Build history of the part. All positions in model axes, mm. Face numbers are marked on the shaded views. A direction names the side the tool comes from. Give positions to 0.01 mm unless a question says otherwise; leave off trailing zeros. Order: outer loops, then holes, each group sorted by start corner. A loop starts at its lowest first (then second) coordinate and runs counter-clockwise, first axis right, second up. Notation, with made-up numbers: M -14.5,54 L -8.5,54 A20 cw -8.5,61 Z; hole C -14,-40 d5. An arc over 180 degrees is marked long. Answer as CSV lines item,"result".
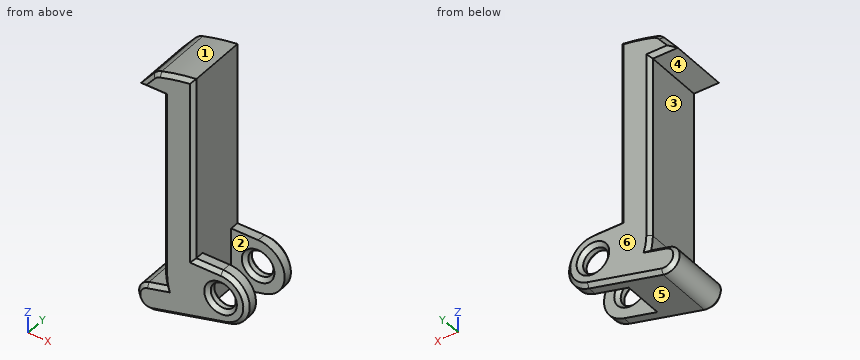
from build123d import *

# Parameters (mm, degrees)
SKETCH1_R           = 1.65
BOSS_EXTRUDE1_DEPTH = 8.6
SKETCH2_W           = 7.05
SKETCH2_H           = 5.3
CUT_EXTRUDE1_DEPTH  = 28.041671481
CHAMFER1_SIZE       = 0.5
CUT_EXTRUDE2_DEPTH  = 36.823034653
FILLET1_R           = 2
CHAMFER2_SIZE       = 0.5


with BuildPart() as part:
    # Sketch1 → Boss-Extrude1 (new body)
    with BuildSketch(Plane(origin=(0, 0, 0), x_dir=(1, 0, 0), z_dir=(0, 1, 0))):
        with BuildLine():
            Line((4.41627224, 31.391101946), (-5.369479089, 33.890916124))
            ThreePointArc((-5.369479089, 33.890916124), (-7.498166182, 32.628501271), (-6.235751329, 30.499814178))
            Line((-6.235751329, 30.499814178), (-3.76509134, 29.868672975))
            ThreePointArc((-3.76509134, 29.868672975), (-3.941042638, 28.941690072), (-4, 28))
            Line((-4, 28), (-4, 4))
            Line((-4, 4), (-7.3, 4))
            Line((-7.3, 4), (-4, 0))
            Line((-4, 0), (0, 0))
            Line((0, 0), (0, 24.5))
            Line((0, 24.5), (3.55, 24.5))
            ThreePointArc((3.55, 24.5), (7.022668773, 27.563454934), (4.41627224, 31.391101946))
        make_face()
        with Locations(Location((3.55, 28, 0), (0, 0, 90))):
            Circle(SKETCH1_R, mode=Mode.SUBTRACT)
    extrude(amount=BOSS_EXTRUDE1_DEPTH)

    # Sketch2 → Cut-Extrude1 (cut, through all)
    with BuildSketch(Plane.XY.offset(-24.5)):
        with Locations((3.525, 4.3)):
            Rectangle(SKETCH2_W, SKETCH2_H)
    extrude(amount=-CUT_EXTRUDE1_DEPTH, mode=Mode.SUBTRACT)

    # Chamfer1
    chamfer1_edges = [part.edges().sort_by_distance(p)[0] for p in [
        (3.55, 0, -26.35),
        (3.55, 8.6, -26.35),
        (3.55, 6.95, -26.35),
        (3.55, 1.65, -26.35),
    ]]
    chamfer(chamfer1_edges, length=CHAMFER1_SIZE)

    # Sketch3 → Cut-Extrude2 (cut, through all)
    with BuildSketch(Plane(origin=(0, 0, 0), x_dir=(1, 0, 0), z_dir=(0, 1, 0))):
        with BuildLine():
            Line((0, 0.225956362), (0, 0))
            Line((0, 0), (-4, 0))
            Line((-4, 0), (-5.140926966, 1.382941776))
            ThreePointArc((-5.140926966, 1.382941776), (-2.597741622, 0.683241903), (0, 0.225956362))
        make_face()
    extrude(amount=CUT_EXTRUDE2_DEPTH, mode=Mode.SUBTRACT)

    # Fillet1
    fillet1_edges = [part.edges().sort_by_distance(p)[0] for p in [
        (-5.140926966, 4.3, -1.382941776),
    ]]
    fillet(fillet1_edges, radius=FILLET1_R)

    # Chamfer2
    chamfer2_edges = [part.edges().sort_by_distance(p)[0] for p in [
        (-5.083597869, 8.6, -1.448008405),
        (-6.409042622, 0, -2.920051663),
        (-5.65, 0, -4),
        (-4, 0, -16),
        (-3.941042638, 0, -28.941690072),
        (7.022668773, 8.6, -27.563454934),
        (-5.000421335, 0, -30.184243577),
        (-7.498166182, 0, -32.628501271),
        (-0.476603424, 0, -32.641009035),
        (7.022668773, 0, -27.563454934),
        (1.775, 0, -24.5),
        (-0.476603424, 8.6, -32.641009035),
        (-7.498166182, 8.6, -32.628501271),
        (-5.000421335, 8.6, -30.184243577),
        (-3.941042638, 8.6, -28.941690072),
        (-4, 8.6, -16),
        (-5.65, 8.6, -4),
        (-6.409042622, 8.6, -2.920051663),
        (0, 0, -12.362978181),
        (0, 8.6, -12.362978181),
        (-2.297358874, 0, -0.617370576),
        (-2.297358874, 8.6, -0.617370576),
        (1.775, 8.6, -24.5),
        (-5.083597869, 0, -1.448008405),
    ]]
    chamfer(chamfer2_edges, length=CHAMFER2_SIZE)


solid = part.part
Item 1: Pull direction Z, two halves, no side cores. Call the marked faces 3, 4, 5 and 6: released by +Z, released by -Z, zero draft, split by the parting line, or undercut.
Geometry says:
face 3,"undercut"
face 4,"undercut"
face 5,"released by -Z"
face 6,"zero draft"
Item 2: Drop flat-ended pins along their axis: pin 1 (1 mm diameter, centred on x = 1.5, y = 1, fed in from +Z); pin 2 (3 mm diameter, centred on x = 3.55, z = -28, fed in from -Y); pin 3 (5 mm diameter, centred on x = -5, y = 3.5, fed in from +Z); pin 4 (4 mm diameter, centred on y = 5, z = -17, fed in from -X). Give the stop position or say it passes through.
Geometry says:
pin 1,"stops at z = -24.5"
pin 2,"passes through"
pin 3,"stops at z = -0.66"
pin 4,"stops at x = -4"
Item 3: Band-saw the part on A-A (z = -4.5). Give the cut face in (x, y).
Geometry says:
outline,"M -4,0.5 L -3.5,0 L -0.5,0 L 0,0.5 L 0,8.1 L -0.5,8.6 L -3.5,8.6 L -4,8.1 Z"
Item 4: Band-saw the part on B-B (y = 5.5). Give the cut face in (x, z), and give its area (3 significant figures).
Geometry says:
outline,"M -7.3,-4 L -4,-4 L -4,-28 A7.55 ccw -3.77,-29.87 L -6.24,-30.5 A1.75 ccw -5.37,-33.89 L 0,-32.52 L 0,-0.23 A28 ccw -4.55,-1.2 A2 ccw -5.52,-1.84 Z"
area,"147 mm2"
Item 5: Probe line 1 along Y through (x, z) = (2, -30.5); line 2 along X through (y, z) = (0.75, -28); line 3 along X through (y, z) = (2.5, -12.5). List the from-to ranges inside material, lowest first. Write a range as from..to.
Geometry says:
line 1,"y = 0..1.65, 6.95..8.6"
line 2,"x = -4..1.9, 5.2..7.05"
line 3,"x = -4..0"
Item 6: 3-axis set-ups, long thin cutter, end or side, ignore diameter. For the marked faces 1 and 2: which of +Z, -Z, +X, -X, +Y, -Y reach the whole face in a straight line?
Geometry says:
face 1,"+Z, -X, +Y, -Y"
face 2,"+Z, -Z, +X"
